```python
from build123d import *
from build123d.topology import SkipClean

# Parameters (mm, degrees)
SKETCH1_R      = 2
EXTRUDE1_DEPTH = 3
EXTRUDE2_START = 3
EXTRUDE2_DEPTH = 3
EXTRUDE3_DEPTH = 2.5


with BuildPart() as part:
    # Sketch1 → Extrude1 (new body)
    with BuildSketch(Plane.XY):
        Circle(SKETCH1_R)
    extrude(amount=EXTRUDE1_DEPTH)

    # Sketch2 → Extrude2 (add)
    with SkipClean():  # the faces are left unmerged after this step: merging them gives an invalid solid
        with BuildSketch(Plane(origin=(0, 0, 0), x_dir=(-1, 0, 0), z_dir=(0, 0, -1)).offset(EXTRUDE2_START)):
            with BuildLine():
                ThreePointArc((-1.732050808, 1), (-1.732050808, -1), (0, -2))
                Line((0, -2), (0, 1))
                Line((0, 1), (-1.732050808, 1))
            make_face()
            with BuildLine():
                Line((0, 1), (0, -2))
                ThreePointArc((0, -2), (1.732050808, -1), (1.732050808, 1))
                Line((1.732050808, 1), (0, 1))
            make_face()
        extrude(amount=-EXTRUDE2_DEPTH)

    # Sketch3 → Extrude3 (cut)
    with SkipClean():  # the faces are left unmerged after this step: merging them gives an invalid solid
        with BuildSketch(Plane.XY.offset(3)):
            with BuildLine():
                ThreePointArc((-1.118033989, 1), (-1.369306394, -0.612372436), (0, -1.5))
                Line((0, -1.5), (0, 1))
                Line((0, 1), (-1.118033989, 1))
            make_face()
            with BuildLine():
                Line((0, 1), (0, -1.5))
                ThreePointArc((0, -1.5), (1.060660172, -1.060660172), (1.5, 0))
                ThreePointArc((1.5, 0), (1.401258538, 0.535233135), (1.118033989, 1))
                Line((1.118033989, 1), (0, 1))
            make_face()
        extrude(amount=-EXTRUDE3_DEPTH, mode=Mode.SUBTRACT)


solid = part.part
```
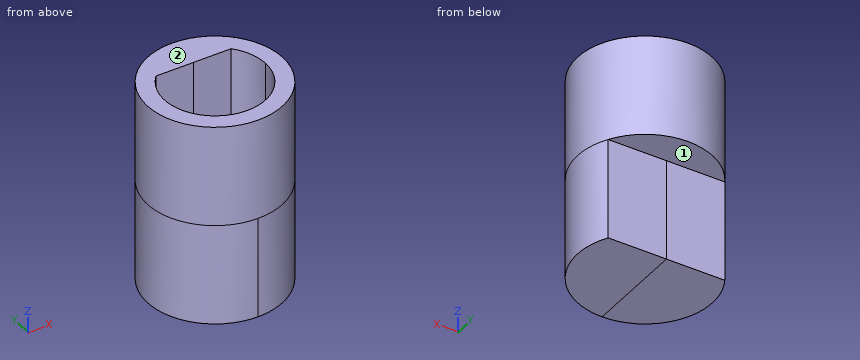
Geometry: final body of the model. Coordinates: model frame, mm. Face numbers are marked on the shaded views. A direction names the side the tool comes from. Round coordinates to 2 decimals unless told otherwise and drop trailing zeros. Order: outer loops, then holes, each group sorted by start corner. A loop starts at its lowest first (then second) coordinate and runs counter-clockwise, first axis right, second up. Notation, with made-up numbers: M -37.5,68 L 2.5,68 A28 cw 2.5,104 Z; hole C -40,-9 d8. An arc over 180 degrees is marked long. One line per item, written item: value.
(1) Pin query (flat end, axial travel): P1, Ø0.5, axis at x = -1, z = -1, coming from the +Y side; P2, Ø0.8, axis at x = 0.5, y = 1.5, coming from the -Z side. Return the tip coordinate at first contact, or that it passes through.
Result sheet:
P1: y = 1
P2: z = 0
(2) Reachability of the marked faces 1 and 2 from +Z, -Z, +X, -X, +Y, -Y: full face, straight path, thin tool, end or side. Return the list, or none.
Result sheet:
face 1: -Z, +X, -X, +Y
face 2: +Z, +X, -X, +Y, -Y
(3) Cut plane A-A (z = 1.5). Return the cut outline in (x, y).
Result sheet:
outline: C 0,0 d4; hole M -1.12,1 A1.5 ccw long 1.12,1 Z
(4) Line query: probe 1 along Z at (x, y) = (0.65, 0.6); probe 2 along X at (y, z) = (0.2, 2.5); probe 3 along Z at (x, y) = (-1.05, 1.5). Output: solid intervals per line, ascending. Write a range as [from, to].
Result sheet:
probe 1: [-3, 0.5]
probe 2: [-1.99, -1.49], [1.49, 1.99]
probe 3: [0, 3]
(5) Cut plane B-B (x = -1.2). Return the cut outline in (y, z).
Result sheet:
outline: M -1.6,-3 L 1,-3 L 1,0 L 1.6,0 L 1.6,3 L 0.9,3 L 0.9,0.5 L -0.9,0.5 L -0.9,3 L -1.6,3 Z
(6) Cut plane D-D (z = -1.15). Return the cut outline in (x, y), and give its area (3 significant figures).
Result sheet:
outline: M -1.73,1 A2 ccw long 1.73,1 Z
area: 10.1 mm2
(7) Cut plane C-C (y = -0.65). Return the cut outline in (x, z), and give its area (3 significant figures).
Result sheet:
outline: M -1.89,-3 L 1.89,-3 L 1.89,3 L 1.35,3 L 1.35,0.5 L -1.35,0.5 L -1.35,3 L -1.89,3 Z
area: 15.9 mm2
